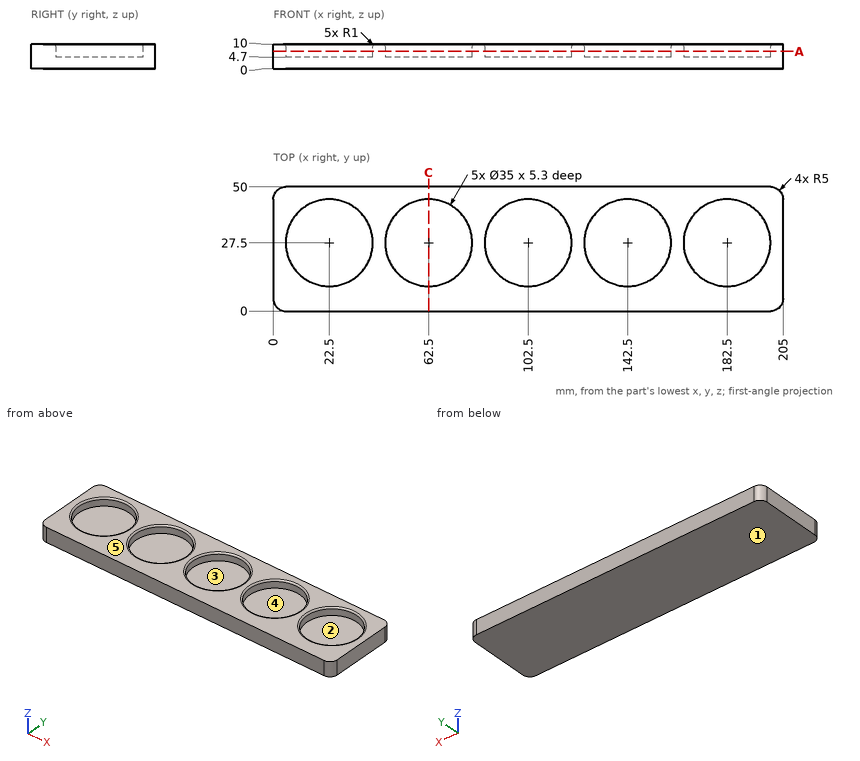
Design review of the part shown in the three views and the two pictorial views. Dimensions are in mm from the part's minimum x, y and z. A direction names the side the tool comes from. Round coordinates to 2 decimals unless told otherwise and drop trailing zeros. Write each loop counter-clockwise with the first axis right and the second up, starting at its lowest first coordinate (ties: lowest second). Pieces come first, ordered by that corner, then holes. Notation, with made-up numbers: (17, 11) -> (71, 11) arc R21 cw to (71, 33) -> close; hole circle Ø4 at (-38.75, 56.25). An arc over 180 degrees is marked (long way). Answer as a JSON object with one key per item and string values.
1. To check wall thickness, follow line 1 along X through (y, z) = (36.5, 7.25); line 2 along Y through (x, z) = (62.5, 6.85); line 3 along X through (y, z) = (42, 5). State the ranges of each line that lie inside material, in increasing order.
Results found:
{"line 1": "x = 0 to 7.49, 37.51 to 47.49, 77.51 to 87.49, 117.51 to 127.49, 157.51 to 167.49, 197.51 to 205", "line 2": "y = 0 to 10, 45 to 50", "line 3": "x = 0 to 12.7, 32.3 to 52.7, 72.3 to 92.7, 112.3 to 132.7, 152.3 to 172.7, 192.3 to 205"}
2. The part is to be moulded in two halves that separate along X. For the marked faces 1, 2 and 3, say which applies: pulls with the +X half, pulls with the -X half, needs draft (parallel to the pull), parting line crosses it, or undercut.
Results found:
{"face 1": "needs draft", "face 2": "undercut", "face 3": "undercut"}
3. We need section C-C on x = 62.5. State the section outline as (y, z) points, and give its area (3 significant figures).
Results found:
{"outline": "(0, 0) -> (50, 0) -> (50, 10) -> (46, 10) arc R1 ccw to (45, 9) -> (45, 4.7) -> (10, 4.7) -> (10, 9) arc R1 ccw to (9, 10) -> (0, 10) -> close", "area": "314 mm^2"}
4. We need section A-A on z = 7. State the section outline as (x, y) points.
Results found:
{"outline": "(0, 5) arc R5 ccw to (5, 0) -> (200, 0) arc R5 ccw to (205, 5) -> (205, 45) arc R5 ccw to (200, 50) -> (5, 50) arc R5 ccw to (0, 45) -> close; hole circle Ø35 at (22.5, 27.5); hole circle Ø35 at (62.5, 27.5); hole circle Ø35 at (102.5, 27.5); hole circle Ø35 at (142.5, 27.5); hole circle Ø35 at (182.5, 27.5)"}
5. Machinability: for the marked faces 4 and 5, which of the approach directions +Z, -Z, +X, -X, +Y, -Y give a long, thin tool a straight path to every point of the face, cutting with its end or side? Answer none if there is none.
Results found:
{"face 4": "+Z", "face 5": "+Z, +X, -X, +Y, -Y"}
6. Clearance check with a flat-ended pin moving along its axis: pin 1 (10.5 mm diameter, centred on x = 174.5, y = 33.5, fed in from +Z). State where the tip first meets the part, or that it passes through.
Results found:
{"pin 1": "stops at z = 4.7"}
